Check sheet for the modelled part. Datum: model origin and axes. Units: mm. Coordinates: 2 decimals unless noted, no trailing zeros. Write each loop counter-clockwise with the first axis right and the second up, starting at its lowest first coordinate (ties: lowest second). Pieces come first, ordered by that corner, then holes. Notation, with made-up numbers: M 69,2.5 L 110,2.5 A22 cw 110,10.5 Z; hole C -23,24.5 d7. An arc over 180 degrees is marked long. Answer as CSV lines item,"result".
from build123d import *

# Parameters (mm, degrees)
SKETCH_W        = 980
SKETCH_H        = 480
PAD_DEPTH       = 1
SKETCH001_R     = 1.8
POCKET_DEPTH    = 1.001
SKETCH030_R     = 2.6
POCKET018_DEPTH = 1.001
POCKET019_DEPTH = 1.001
POCKET022_DEPTH = 1.001


with BuildPart() as part:
    # Sketch → Pad (new body)
    with BuildSketch(Plane.XY):
        Rectangle(SKETCH_W, SKETCH_H)
    extrude(amount=PAD_DEPTH)

    # Sketch001 (on Face6 of Pad) → Pocket (cut, through all)
    with BuildSketch(Plane.XY.offset(1)):
        with Locations((0, 232.5)):
            Circle(SKETCH001_R)
        with Locations((156, 232.5)):
            Circle(SKETCH001_R)
        with Locations((312, 232.5)):
            Circle(SKETCH001_R)
        with Locations((468, 232.5)):
            Circle(SKETCH001_R)
        with Locations((-156, 232.5)):
            Circle(SKETCH001_R)
        with Locations((-312, 232.5)):
            Circle(SKETCH001_R)
        with Locations((-468, 232.5)):
            Circle(SKETCH001_R)
        with Locations((482.5, 73)):
            Circle(SKETCH001_R)
        with Locations((482.5, 218)):
            Circle(SKETCH001_R)
        with Locations((-482.5, 218)):
            Circle(SKETCH001_R)
        with Locations((-482.5, 73)):
            Circle(SKETCH001_R)
        with Locations((-468, -232.5)):
            Circle(SKETCH001_R)
        with Locations((-312, -232.5)):
            Circle(SKETCH001_R)
        with Locations((-156, -232.5)):
            Circle(SKETCH001_R)
        with Locations((0, -232.5)):
            Circle(SKETCH001_R)
        with Locations((156, -232.5)):
            Circle(SKETCH001_R)
        with Locations((312, -232.5)):
            Circle(SKETCH001_R)
        with Locations((468, -232.5)):
            Circle(SKETCH001_R)
        with Locations((482.5, -218)):
            Circle(SKETCH001_R)
        with Locations((-482.5, -218)):
            Circle(SKETCH001_R)
        with Locations((482.5, -73)):
            Circle(SKETCH001_R)
        with Locations((-482.5, -73)):
            Circle(SKETCH001_R)
    extrude(amount=-POCKET_DEPTH, mode=Mode.SUBTRACT)

    # Sketch030 → Pocket018 (cut, through all)
    with BuildSketch(Plane.XY.offset(1)):
        with Locations((320.499908, -56.500045)):
            Circle(SKETCH030_R)
        with Locations((433.499908, -56.500045)):
            Circle(SKETCH030_R)
        with Locations((320.499908, 56.499955)):
            Circle(SKETCH030_R)
        with Locations((433.499908, 56.499955)):
            Circle(SKETCH030_R)
    extrude(amount=-POCKET018_DEPTH, mode=Mode.SUBTRACT)

    # Sketch029 (on Face5 of Pocket) → Pocket019 (cut, through all)
    with BuildSketch(Plane.XY.offset(1)):
        with BuildLine():
            ThreePointArc((326.999908, 54.999955), (323.464375, 53.535489), (321.999908, 49.999955))
            Line((321.999908, -50.000045), (321.999908, 49.999955))
            ThreePointArc((321.999908, -50.000045), (323.464375, -53.535579), (326.999908, -55.000045))
            Line((326.999908, -55.000045), (426.999908, -55.000045))
            ThreePointArc((426.999908, -55.000045), (430.535442, -53.535579), (431.999908, -50.000045))
            Line((431.999908, -50.000045), (431.999908, 49.999955))
            ThreePointArc((431.999908, 49.999955), (430.535442, 53.535489), (426.999908, 54.999955))
            Line((326.999908, 54.999955), (426.999908, 54.999955))
        make_face()
    extrude(amount=-POCKET019_DEPTH, mode=Mode.SUBTRACT)

    # Sketch037 (on Face5 of Pocket019) → Pocket022 (cut, through all)
    with BuildSketch(Plane.XY.offset(1)):
        with BuildLine():
            ThreePointArc((232, 190), (240, 182), (248, 190))
            Line((248, 190), (248, 198))
            ThreePointArc((248, 198), (240, 206), (232, 198))
            Line((232, 190), (232, 198))
        make_face()
        with BuildLine():
            Line((-232, 190), (-232, 198))
            ThreePointArc((-232, 198), (-240, 206), (-248, 198))
            Line((-248, 190), (-248, 198))
            ThreePointArc((-248, 190), (-240, 182), (-232, 190))
        make_face()
    extrude(amount=-POCKET022_DEPTH, mode=Mode.SUBTRACT)


solid = part.part
1) Depth check by flat-ended pin: P1, Ø4, axis at x = 482.5, y = -73, coming from the -Z side; P2, Ø4, axis at x = 433.5, y = 56.5, coming from the -Z side. Enter the tip coordinate at first touch or a pass-through.
Answer key:
P1,"stops at z = 0"
P2,"passes through"
2) Thickness scan on line 1 along Y through (x, z) = (156, 0.6); line 2 along X through (y, z) = (205, 0.2); line 3 along Y through (x, z) = (-239.5, 0.5). Record the ranges inside material, lowest first.
Answer key:
line 1,"y = -240 to -234.3, -230.7 to 230.7, 234.3 to 240"
line 2,"x = -490 to -243.87, -236.13 to 236.13, 243.87 to 490"
line 3,"y = -240 to 182.02, 205.98 to 240"
3) Section check A-A, the plane y = 37. Record the boundary of the cut face in (x, z), plus the area to 3 significant figures.
Answer key:
outline,"M -490,0 L 322,0 L 322,1 L -490,1 Z; M 432,0 L 490,0 L 490,1 L 432,1 Z"
area,"870 mm2"
4) Section check B-B, the plane z = 0.45. Give the number of separate pieces and of enclosed holes in the cut face, plus the area to 3 significant figures.
Answer key:
separate pieces,"1"
enclosed holes,"29"
area,"457,000 mm2"
